```python
from build123d import *

# Parameters (mm, degrees)
SKETCH1_W           = 330.2
SKETCH1_H           = 31.75
SKETCH1_R           = 7.19455
BOSS_EXTRUDE1_DEPTH = 2.159
SKETCH2_R           = 20.6375
SKETCH2_R_2         = 7.19455
BOSS_EXTRUDE2_DEPTH = 4.318
FILLET1_R           = 457.2
BOSS_EXTRUDE3_DEPTH = 4.318
CUT_EXTRUDE2_DEPTH  = 5.318


with BuildPart() as part:
    # Sketch1 → Boss-Extrude1 (new body, symmetric)
    with BuildSketch(Plane(origin=(0, 0, 0), x_dir=(1, 0, 0), z_dir=(0, 1, 0))):
        Rectangle(SKETCH1_W, SKETCH1_H)
        Circle(SKETCH1_R, mode=Mode.SUBTRACT)
    extrude(amount=BOSS_EXTRUDE1_DEPTH, both=True)

    # Sketch2 → Boss-Extrude2 (add)
    with BuildSketch(Plane(origin=(0, 2.159, 0), x_dir=(1, 0, 0), z_dir=(0, 1, 0))):
        Circle(SKETCH2_R)
        Circle(SKETCH2_R_2, mode=Mode.SUBTRACT)
    extrude(amount=-BOSS_EXTRUDE2_DEPTH)

    # Fillet1
    fillet1_edges = [part.edges().sort_by_distance(p)[0] for p in [
        (13.186765382, 0, 15.875),
        (-13.186765382, 0, 15.875),
        (13.186765382, 0, -15.875),
        (-13.186765382, 0, -15.875),
    ]]
    fillet(fillet1_edges, radius=FILLET1_R)

    # Sketch5 → Boss-Extrude3 (add)
    with BuildSketch(Plane.XZ.offset(2.159)):
        Polygon((-165.1, 15.875), (-165.1, 22.225), (-164.465, 22.225), (-160.3375, 19.05), (-130.175, 15.875), align=None)
        Polygon((165.1, -15.875), (165.1, -22.225), (164.465, -22.225), (160.3375, -19.05), (130.175, -15.875), align=None)
    extrude(amount=-BOSS_EXTRUDE3_DEPTH)

    # Sketch7 → Cut-Extrude2 (cut, through all)
    with BuildSketch(Plane.XZ.offset(2.159)):
        with BuildLine():
            Line((164.335006542, 15.875), (165.1, 15.875))
            Line((165.1, 15.875), (165.1, 0))
            ThreePointArc((165.1, 0), (164.908640738, 7.94671064), (164.335006542, 15.875))
        make_face()
        with BuildLine():
            Line((-164.335006542, -15.875), (-165.1, -15.875))
            Line((-165.1, -15.875), (-165.1, 0))
            ThreePointArc((-165.1, 0), (-164.908640738, -7.94671064), (-164.335006542, -15.875))
        make_face()
    extrude(amount=-CUT_EXTRUDE2_DEPTH, mode=Mode.SUBTRACT)


solid = part.part
```
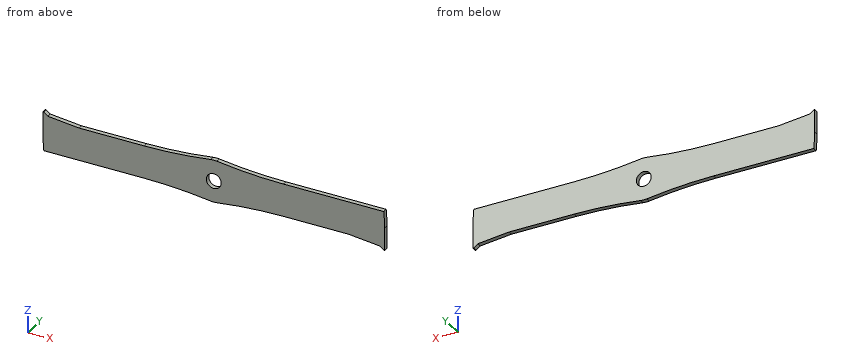
Part model, mm, in its own coordinate system. Coordinates: 2 decimals unless noted, no trailing zeros. Order: outer loops, then holes, each group sorted by start corner. A loop starts at its lowest first (then second) coordinate and runs counter-clockwise, first axis right, second up. Notation, with made-up numbers: (10, 78) - (51, 78) arc R16 ccw to (51, 83) - close; hole circle Ø11 at (57, -16.5). An arc over 180 degrees is marked (long way). Return JSON: item names as keys, results as strings. Group by question number.
Item 1: Cut at B-B (x = 0). List the corners of the cut face in (y, z).
Item 2: Drill centre lines: probe 1 along X at (y, z) = (1, 0); probe 2 along X at (y, z) = (-1.3, -2.5); probe 3 along Z at (x, y) = (101, 1.4) (3 decimals). Where is each one in solid material? Low to high. Write a range as from..to.
Item 3: Cut at C-C (x = 136). List the corners of the cut face in (y, z) (3 decimals).
Item 4: Pin check, flat tips, straight feed: pin 1 (2 mm diameter, centred on x = 96, y = -1, fed in from -Z) (3 decimals); pin 2 (1.3 mm diameter, centred on x = 139, y = 1, fed in from +Z) (3 decimals); pin 3 (1.5 mm diameter, centred on y = 0.5, z = -12, fed in from -X). Stop position of each tip, or through.
Item 5: Cut at D-D (x = 57.5). List the corners of the cut face in (y, z), plus the area to 3 significant figures.
Check values:
{
 "1": {"outline": "(-2.16, -20.64) - (2.16, -20.64) - (2.16, -7.19) - (-2.16, -7.19) - close; (-2.16, 7.19) - (2.16, 7.19) - (2.16, 20.64) - (-2.16, 20.64) - close"},
 "2": {"probe 1": "x = -165.1..-7.19, 7.19..165.1", "probe 2": "x = -165.08..-6.75, 6.75..165.1", "probe 3": "z = -15.875..15.875"},
 "3": {"outline": "(-2.159, -16.488) - (2.159, -16.488) - (2.159, 15.875) - (-2.159, 15.875) - close"},
 "4": {"pin 1": "stops at z = -15.875", "pin 2": "stops at z = 15.875", "pin 3": "stops at x = -164.72"},
 "5": {"outline": "(-2.16, -15.98) - (2.16, -15.98) - (2.16, 15.98) - (-2.16, 15.98) - close", "area": "138 mm2"}
}
